from build123d import *

# Parameters (mm, degrees)
F0_R     = 12.7
F1_DEPTH = 25.4
F2_R     = 12.7
F3_DEPTH = 25.4
F4_R     = 12.7


with BuildPart() as f1:
    # F0 (on Front) → F1 (new body)
    with BuildSketch(Plane.XZ):
        with BuildLine():
            Line((59.5375982285, 0), (-27.8245286434, 59.1343283417))
            ThreePointArc((-27.8245286434, 59.1343283417), (-53.9686611032, 60.5365993129), (-67.4624017715, 38.1))
            Line((-67.4624017715, 38.1), (-67.4624017715, -12.7))
            Line((-67.4624017715, -12.7), (59.5375982285, -12.7))
            Line((59.5375982285, -12.7), (59.5375982285, 0))
        make_face()
        with Locations((-42.0624017715, 38.1)):
            Circle(F0_R, mode=Mode.SUBTRACT)
    extrude(amount=F1_DEPTH)

    # F2 (on face) → F3 (join)
    with BuildSketch(Plane.XZ.offset(25.4)):
        with BuildLine():
            Line((-16.6746217208, 0), (-16.6746217208, 37.3122030112))
            Line((-16.6746217208, 37.3122030112), (-16.6746217208, 38.8877969888))
            ThreePointArc((-16.6746217208, 38.8877969888), (-19.8131634606, 50.352811701), (-27.8245286434, 59.1343283417))
            ThreePointArc((-27.8245286434, 59.1343283417), (-53.9686611032, 60.5365993129), (-67.4624017715, 38.1))
            Line((-67.4624017715, 38.1), (-67.4624017715, 0))
            Line((-67.4624017715, 0), (-67.4624017715, -12.7))
            Line((-67.4624017715, -12.7), (59.5375982285, -12.7))
            Line((59.5375982285, -12.7), (59.5375982285, 0))
            Line((59.5375982285, 0), (-16.6746217208, 0))
        make_face()
        with Locations((-42.0624017715, 38.1)):
            Circle(F2_R, mode=Mode.SUBTRACT)
    extrude(amount=F3_DEPTH)

    # F4
    f4_edges = [f1.edges().sort_by_distance(p)[0] for p in [
        (59.537598, -50.8, -6.35),
    ]]
    fillet(f4_edges, radius=F4_R)


solid = f1.part
Read the model definition and answer for the solid it produces. Units are mm, in the model's axes. A direction names the side the tool comes from. Coordinates: 2 decimals unless noted, no trailing zeros. Loops run counter-clockwise (first coordinate to the right, second up) from the corner with the lowest first, then second, coordinate; pieces in that order, holes last. Notation, with made-up numbers: (-1.5, 70) -> (56.5, 70) arc R32 ccw to (56.5, 99) -> close; hole circle Ø11 at (42, -13.5). An arc over 180 degrees is marked (long way). Answer in a Markdown table with one row per item.
Item 1: A cutting plane is placed at B-B on x = -39.5. Determine the outline of the cut face in (y, z), plus the area to 3 significant figures.
Returned:
| item | result |
|---|---|
| outline | (-50.8, -12.7) -> (0, -12.7) -> (0, 25.66) -> (-50.8, 25.66) -> close; (-50.8, 50.54) -> (0, 50.54) -> (0, 63.37) -> (-50.8, 63.37) -> close |
| area | 2,600 mm^2 |
Item 2: Straight lines are drawn through the part: line 1 along X through (y, z) = (-28, 38); line 2 along Y through (x, z) = (5, 21); line 3 along Z through (x, y) = (-53, -47). For each, find the intervals that lie inside material, in ascending order. Write a range as [from, to].
Returned:
| item | result |
|---|---|
| line 1 | x = [-67.46, -54.76], [-29.36, -16.67] |
| line 2 | y = [-25.4, 0] |
| line 3 | z = [-12.7, 31.65], [44.55, 61.02] |
Item 3: A cutting plane is placed at C-C on z = 11.5. Determine the outline of the cut face in (x, y), plus the area to 3 significant figures.
Returned:
| item | result |
|---|---|
| outline | (-67.46, -50.8) -> (-16.67, -50.8) -> (-16.67, -25.4) -> (42.55, -25.4) -> (42.55, 0) -> (-67.46, 0) -> close |
| area | 4,080 mm^2 |
Item 4: A cutting plane is placed at D-D on y = -41. Determine the outline of the cut face in (x, z).
Returned:
| item | result |
|---|---|
| outline | (-67.46, -12.7) -> (59.2, -12.7) -> (59.2, 0) -> (-16.67, 0) -> (-16.67, 38.89) arc R25.4 ccw to (-67.46, 38.1) -> close; hole circle Ø25.4 at (-42.06, 38.1) |
Item 5: For faces 1 (the cylindrical face through (-51.423, -25.044, 46.683)), 2 (the flat face through (9, -25.4, 19)), determine the directions among +Z, -Z, +X, -X, +Y, -Y from which every point of the face is accessible in a straight line to the end or side of a thin tool.
Returned:
| item | result |
|---|---|
| face 1 | +Y, -Y |
| face 2 | +Z, +X, -Y |
Item 6: Each of these flat-tipped pins is pushed along its axis until it touches: P1, Ø12.5, axis at x = 3.5, y = -39.5, coming from the +Z side; P2, Ø4, axis at y = -29, z = 8.5, coming from the +X side; P3, Ø12, axis at x = 24, y = -11, coming from the +Z side. Where does it stop, or does it pass through?
Returned:
| item | result |
|---|---|
| P1 | stops at z = 0 |
| P2 | stops at x = -16.67 |
| P3 | stops at z = 28.12 |
Item 7: A cutting plane is placed at A-A on y = -31. Determine the outline of the cut face in (x, z), plus the area to 3 significant figures.
Returned:
| item | result |
|---|---|
| outline | (-67.46, -12.7) -> (59.54, -12.7) -> (59.54, 0) -> (-16.67, 0) -> (-16.67, 38.89) arc R25.4 ccw to (-67.46, 38.1) -> close; hole circle Ø25.4 at (-42.06, 38.1) |
| area | 4,050 mm^2 |
